from build123d import *

# Parameters (mm, degrees)
SKETCH_1_W          = 4.708553468
SKETCH_1_H          = 29.97466091
EXTRUDE_1_DEPTH     = 4.1
EXTRUDE_1_2_DEPTH   = 4.1
SKETCH_2_W          = 4.708553468
SKETCH_2_H          = 29.97466091
EXTRUDE_2_DEPTH     = 9
SKETCH_3_W          = 6
SKETCH_3_H          = 29.97466091
EXTRUDE_3_DEPTH     = 32.057569214
SKETCH_6_R          = 1
EXTRUDE_4_DEPTH     = 3
SKETCH_7_R          = 1.5
EXTRUDE_5_DEPTH     = 0.5
CUT_EXTRUDE_1_REACH = 33.926
SKETCH_9_W          = 32.057569214
SKETCH_9_H          = 5.97466091
EXTRUDE_6_DEPTH     = 2
SKETCH_12_W         = 4.708553468
SKETCH_12_H         = 13.1
EXTRUDE_7_DEPTH     = 2
SKETCH_13_W         = 32.057569214
SKETCH_13_H         = 6
CUT_EXTRUDE_3_DEPTH = 6.8
CUT_EXTRUDE_4_REACH = 35.242
SKETCH_14_W         = 3.528784607
SKETCH_14_H         = 10.5
CHAMFER_1_SIZE      = 2
CHAMFER_2_SIZE      = 0.5
CUT_EXTRUDE_5_REACH = 44.936
SKETCH_15_W         = 0.5
SKETCH_15_H         = 1
CHAMFER_3_SIZE      = 0.2
CHAMFER_4_SIZE      = 0.2
SKETCH_16_W         = 32.057569214
SKETCH_16_H         = 2
EXTRUDE_8_DEPTH     = 13.1
CUT_EXTRUDE_7_REACH = 43.372
SKETCH_18_W         = 32.057569214
SKETCH_18_H         = 2
EXTRUDE_9_DEPTH     = 7.1
CUT_EXTRUDE_8_DEPTH = 4


with BuildPart() as part:
    # Sketch 1 → Extrude 1 (new body)
    with BuildSketch(Plane.XY):
        with Locations((-18.383061341, 5.449009398)):
            Rectangle(SKETCH_1_W, SKETCH_1_H)
    extrude(amount=EXTRUDE_1_DEPTH)



with BuildPart() as body_2:
    # Sketch 1 → Extrude 1 2 (new body)
    with BuildSketch(Plane.XY):
        with Locations((18.383061341, 5.449009398)):
            Rectangle(SKETCH_1_W, SKETCH_1_H)
    extrude(amount=EXTRUDE_1_2_DEPTH)


with BuildPart() as part_1:
    add(part.part)

    add(body_2.part)  # Extrude 2 merges body 2
    # Sketch 2 → Extrude 2 (add)
    with BuildSketch(Plane.XY.offset(4.1)):
        with Locations((-18.383061341, 5.449009398)):
            Rectangle(SKETCH_2_W, SKETCH_2_H)
        with Locations((18.383061341, 5.449009398)):
            Rectangle(SKETCH_2_W, SKETCH_2_H)
    extrude(amount=EXTRUDE_2_DEPTH)

    # Sketch 3 → Extrude 3 (add)
    with BuildSketch(Plane.ZY.offset(-16.028784607)):
        with Locations((10.1, 5.449009398)):
            Rectangle(SKETCH_3_W, SKETCH_3_H)
    extrude(amount=EXTRUDE_3_DEPTH)

    # Sketch 6 → Extrude 4 (add)
    with BuildSketch(Plane.XY.offset(13.1)):
        with Locations((-10.5, 5.961678943)):
            Circle(SKETCH_6_R)
        with Locations((10.5, -7.538321057)):
            Circle(SKETCH_6_R)
        with Locations((-10.5, -7.538321057)):
            Circle(SKETCH_6_R)
        with Locations((10.5, 5.961678943)):
            Circle(SKETCH_6_R)
    extrude(amount=EXTRUDE_4_DEPTH)

    # Sketch 7 → Extrude 5 (add)
    with BuildSketch(Plane.XY.offset(13.1)):
        with Locations((-10.5, 5.961678943)):
            Circle(SKETCH_7_R)
        with Locations((-10.5, -7.538321057)):
            Circle(SKETCH_7_R)
        with Locations(Location((10.5, -7.538321057, 0), (0, 0, 180))):
            Circle(SKETCH_7_R)
        with Locations(Location((10.5, 5.961678943, 0), (0, 0, 180))):
            Circle(SKETCH_7_R)
    extrude(amount=EXTRUDE_5_DEPTH)

    # Sketch 9 → Cut-Extrude 1 (cut, up to next)
    with BuildSketch(Plane.XY.offset(13.1), mode=Mode.PRIVATE) as cut_extrude_1_sk1:
        with Locations((0, 17.449009398)):
            Rectangle(SKETCH_9_W, SKETCH_9_H)
    cut_extrude_1_tool1 = extrude(cut_extrude_1_sk1.sketch, amount=-CUT_EXTRUDE_1_REACH, mode=Mode.PRIVATE) & part_1.part
    add(cut_extrude_1_tool1.solids().sort_by_distance((0, 17.449009, 13.1))[0], mode=Mode.SUBTRACT)

    # Sketch 11 → Extrude 6 (add)
    with BuildSketch(Plane.XZ.offset(9.538321057)):
        Polygon((-20.737338075, 0), (-16.028784607, 0), (-16.028784607, 7.1), (16.028784607, 7.1), (16.028784607, 0), (20.737338075, 0), (20.737338075, 13.1), (-20.737338075, 13.1), align=None)
    extrude(amount=EXTRUDE_6_DEPTH)

    # Sketch 12 → Extrude 7 (add)
    with BuildSketch(Plane(origin=(0, 20.436339853, 0), x_dir=(1, 0, 0), z_dir=(0, 1, 0))):
        with Locations((18.383061341, -6.55)):
            Rectangle(SKETCH_12_W, SKETCH_12_H)
        with Locations((-18.383061341, -6.55)):
            Rectangle(SKETCH_12_W, SKETCH_12_H)
    extrude(amount=EXTRUDE_7_DEPTH)

    # Sketch 13 → Cut-Extrude 3 (cut)
    with BuildSketch(Plane(origin=(0, 14.461678943, 0), x_dir=(1, 0, 0), z_dir=(0, 1, 0))):
        with Locations((0, -10.1)):
            Rectangle(SKETCH_13_W, SKETCH_13_H)
    extrude(amount=-CUT_EXTRUDE_3_DEPTH, mode=Mode.SUBTRACT)

    # Sketch 14 → Cut-Extrude 4 (cut, up to next)
    with BuildSketch(Plane.XY.offset(13.1), mode=Mode.PRIVATE) as cut_extrude_4_sk1:
        with Locations((-14.264392304, -0.788321057)):
            Rectangle(SKETCH_14_W, SKETCH_14_H)
    cut_extrude_4_tool1 = extrude(cut_extrude_4_sk1.sketch, amount=-CUT_EXTRUDE_4_REACH, mode=Mode.PRIVATE) & part_1.part
    # Sketch 14 → Cut-Extrude 4 (cut, up to next)
    with BuildSketch(Plane.XY.offset(13.1), mode=Mode.PRIVATE) as cut_extrude_4_sk2:
        with Locations((14.264392304, -0.788321057)):
            Rectangle(SKETCH_14_W, SKETCH_14_H)
    cut_extrude_4_tool2 = extrude(cut_extrude_4_sk2.sketch, amount=-CUT_EXTRUDE_4_REACH, mode=Mode.PRIVATE) & part_1.part
    add(cut_extrude_4_tool1.solids().sort_by_distance((-14.264392, -0.788321, 13.1))[0], mode=Mode.SUBTRACT)
    add(cut_extrude_4_tool2.solids().sort_by_distance((14.264392, -0.788321, 13.1))[0], mode=Mode.SUBTRACT)

    # Chamfer 1
    chamfer_1_edges = [part_1.edges().sort_by_distance(p)[0] for p in [
        (-20.737338075, 5.449009398, 13.1),
        (20.737338075, 5.449009398, 13.1),
    ]]
    chamfer(chamfer_1_edges, length=CHAMFER_1_SIZE)

    # Chamfer 2
    chamfer_2_edges = [part_1.edges().sort_by_distance(p)[0] for p in [
        (16.028784607, 7.661678943, 10.1),
        (-16.028784607, 7.661678943, 10.1),
        (-16.028784607, -6.038321057, 10.1),
        (-12.5, 4.461678943, 10.1),
        (-12.5, -6.038321057, 10.1),
        (-16.028784607, 4.461678943, 10.1),
        (16.028784607, 4.461678943, 10.1),
        (12.5, 4.461678943, 10.1),
        (16.028784607, -6.038321057, 10.1),
        (12.5, -6.038321057, 10.1),
    ]]
    chamfer(chamfer_2_edges, length=CHAMFER_2_SIZE)

    # Sketch 15 → Cut-Extrude 5 (cut, up to next)
    with BuildSketch(Plane.XZ.offset(11.538321057), mode=Mode.PRIVATE) as cut_extrude_5_sk1:
        with Locations((-20.487338075, 5.05)):
            Rectangle(SKETCH_15_W, SKETCH_15_H)
    cut_extrude_5_tool1 = extrude(cut_extrude_5_sk1.sketch, amount=-CUT_EXTRUDE_5_REACH, mode=Mode.PRIVATE) & part_1.part
    # Sketch 15 → Cut-Extrude 5 (cut, up to next)
    with BuildSketch(Plane.XZ.offset(11.538321057), mode=Mode.PRIVATE) as cut_extrude_5_sk2:
        with Locations((-20.487338075, 3.55)):
            Rectangle(SKETCH_15_W, SKETCH_15_H)
    cut_extrude_5_tool2 = extrude(cut_extrude_5_sk2.sketch, amount=-CUT_EXTRUDE_5_REACH, mode=Mode.PRIVATE) & part_1.part
    # Sketch 15 → Cut-Extrude 5 (cut, up to next)
    with BuildSketch(Plane.XZ.offset(11.538321057), mode=Mode.PRIVATE) as cut_extrude_5_sk3:
        with Locations((-20.487338075, 2.05)):
            Rectangle(SKETCH_15_W, SKETCH_15_H)
    cut_extrude_5_tool3 = extrude(cut_extrude_5_sk3.sketch, amount=-CUT_EXTRUDE_5_REACH, mode=Mode.PRIVATE) & part_1.part
    # Sketch 15 → Cut-Extrude 5 (cut, up to next)
    with BuildSketch(Plane.XZ.offset(11.538321057), mode=Mode.PRIVATE) as cut_extrude_5_sk4:
        with Locations((-20.487338075, 6.55)):
            Rectangle(SKETCH_15_W, SKETCH_15_H)
    cut_extrude_5_tool4 = extrude(cut_extrude_5_sk4.sketch, amount=-CUT_EXTRUDE_5_REACH, mode=Mode.PRIVATE) & part_1.part
    # Sketch 15 → Cut-Extrude 5 (cut, up to next)
    with BuildSketch(Plane.XZ.offset(11.538321057), mode=Mode.PRIVATE) as cut_extrude_5_sk5:
        with Locations((20.487338075, 5.55)):
            Rectangle(SKETCH_15_W, SKETCH_15_H)
    cut_extrude_5_tool5 = extrude(cut_extrude_5_sk5.sketch, amount=-CUT_EXTRUDE_5_REACH, mode=Mode.PRIVATE) & part_1.part
    # Sketch 15 → Cut-Extrude 5 (cut, up to next)
    with BuildSketch(Plane.XZ.offset(11.538321057), mode=Mode.PRIVATE) as cut_extrude_5_sk6:
        with Locations((20.487338075, 1.05)):
            Rectangle(SKETCH_15_W, SKETCH_15_H)
    cut_extrude_5_tool6 = extrude(cut_extrude_5_sk6.sketch, amount=-CUT_EXTRUDE_5_REACH, mode=Mode.PRIVATE) & part_1.part
    # Sketch 15 → Cut-Extrude 5 (cut, up to next)
    with BuildSketch(Plane.XZ.offset(11.538321057), mode=Mode.PRIVATE) as cut_extrude_5_sk7:
        with Locations((20.487338075, 2.55)):
            Rectangle(SKETCH_15_W, SKETCH_15_H)
    cut_extrude_5_tool7 = extrude(cut_extrude_5_sk7.sketch, amount=-CUT_EXTRUDE_5_REACH, mode=Mode.PRIVATE) & part_1.part
    # Sketch 15 → Cut-Extrude 5 (cut, up to next)
    with BuildSketch(Plane.XZ.offset(11.538321057), mode=Mode.PRIVATE) as cut_extrude_5_sk8:
        with Locations((20.487338075, 4.05)):
            Rectangle(SKETCH_15_W, SKETCH_15_H)
    cut_extrude_5_tool8 = extrude(cut_extrude_5_sk8.sketch, amount=-CUT_EXTRUDE_5_REACH, mode=Mode.PRIVATE) & part_1.part
    add(cut_extrude_5_tool1.solids().sort_by_distance((-20.487338, -11.538321, 5.05))[0], mode=Mode.SUBTRACT)
    add(cut_extrude_5_tool2.solids().sort_by_distance((-20.487338, -11.538321, 3.55))[0], mode=Mode.SUBTRACT)
    add(cut_extrude_5_tool3.solids().sort_by_distance((-20.487338, -11.538321, 2.05))[0], mode=Mode.SUBTRACT)
    add(cut_extrude_5_tool4.solids().sort_by_distance((-20.487338, -11.538321, 6.55))[0], mode=Mode.SUBTRACT)
    add(cut_extrude_5_tool5.solids().sort_by_distance((20.487338, -11.538321, 5.55))[0], mode=Mode.SUBTRACT)
    add(cut_extrude_5_tool6.solids().sort_by_distance((20.487338, -11.538321, 1.05))[0], mode=Mode.SUBTRACT)
    add(cut_extrude_5_tool7.solids().sort_by_distance((20.487338, -11.538321, 2.55))[0], mode=Mode.SUBTRACT)
    add(cut_extrude_5_tool8.solids().sort_by_distance((20.487338, -11.538321, 4.05))[0], mode=Mode.SUBTRACT)

    # Chamfer 3
    chamfer_3_edges = [part_1.edges().sort_by_distance(p)[0] for p in [
        (-20.237338075, 5.449009398, 4.05),
        (-20.237338075, 5.449009398, 3.05),
        (-20.237338075, 5.449009398, 2.55),
        (-20.237338075, 5.449009398, 1.55),
        (-20.237338075, 5.449009398, 7.05),
        (-20.237338075, 5.449009398, 6.05),
        (-20.237338075, 5.449009398, 5.55),
        (-20.237338075, 5.449009398, 4.55),
    ]]
    chamfer(chamfer_3_edges, length=CHAMFER_3_SIZE)

    # Chamfer 4
    chamfer_4_edges = [part_1.edges().sort_by_distance(p)[0] for p in [
        (20.237338075, 5.449009398, 6.05),
        (20.237338075, 5.449009398, 5.05),
        (20.237338075, 5.449009398, 1.55),
        (20.237338075, 5.449009398, 0.55),
        (20.237338075, 5.449009398, 3.05),
        (20.237338075, 5.449009398, 2.05),
        (20.237338075, 5.449009398, 4.55),
        (20.237338075, 5.449009398, 3.55),
    ]]
    chamfer(chamfer_4_edges, length=CHAMFER_4_SIZE)

    # Sketch 16 → Extrude 8 (add)
    with BuildSketch(Plane(origin=(0, 0, 0), x_dir=(-1, 0, 0), z_dir=(0, 0, -1))):
        with Locations((0, 21.436339853)):
            Rectangle(SKETCH_16_W, SKETCH_16_H)
    extrude(amount=-EXTRUDE_8_DEPTH)

    # Sketch 17 → Cut-Extrude 7 (cut, up to next)
    with BuildSketch(Plane.XZ.offset(-20.436339853), mode=Mode.PRIVATE) as cut_extrude_7_sk1:
        with BuildLine():
            Line((4.465561881, 1.229756424), (4.470622966, 1.343469934))
            Line((4.470622966, 1.343469934), (4.470622966, 1.943469934))
            add(Edge.make_bspline(
                [(4.470622966, 1.943469934), (4.470622966, 3.223469934), (3.190622966, 3.223469934)],
                knots=[1.814608209, 1.814608209, 1.814608209, 3.385404536, 3.385404536, 3.385404536], degree=2, weights=[1, 0.707106781, 1]))
            Line((3.190622966, 3.223469934), (-3.189377034, 3.223469934))
            ThreePointArc((-3.189377034, 3.223469934), (-4.094473714, 2.848566614), (-4.469377034, 1.943469934))
            Line((-4.469377034, 1.943469934), (-4.469377034, 1.343469934))
            Line((-4.469377034, 1.343469934), (-4.489171494, 5.5e-08))
            Line((-4.489171494, 5.5e-08), (4.410828707, 4e-09))
            Line((4.410828707, 4e-09), (4.465561881, 1.229756424))
        make_face()
    cut_extrude_7_tool1 = extrude(cut_extrude_7_sk1.sketch, amount=-CUT_EXTRUDE_7_REACH, mode=Mode.PRIVATE) & part_1.part
    add(cut_extrude_7_tool1.solids().sort_by_distance((-0.00786, 20.43634, 1.579655))[0], mode=Mode.SUBTRACT)

    # Sketch 18 → Extrude 9 (add)
    with BuildSketch(Plane(origin=(0, 0, 7.1), x_dir=(-1, 0, 0), z_dir=(0, 0, -1))):
        with Locations((0, -10.538321057)):
            Rectangle(SKETCH_18_W, SKETCH_18_H)
    extrude(amount=EXTRUDE_9_DEPTH)

    # Sketch 19 → Cut-Extrude 8 (cut)
    with BuildSketch(Plane(origin=(0, 0, 7.1), x_dir=(-1, 0, 0), z_dir=(0, 0, -1))):
        Polygon((-16.028784607, -5.538321057), (-16.028784607, -9.538321057), (16.028784607, -9.538321057), (16.028784607, -5.538321057), (15.528784607, -6.038321057), (13, -6.038321057), (12.5, -5.538321057), (12.5, 3.961678943), (13, 4.461678943), (15.528784607, 4.461678943), (16.028784607, 3.961678943), (16.028784607, 8.161678943), (15.528784607, 7.661678943), (-15.528784607, 7.661678943), (-16.028784607, 8.161678943), (-16.028784607, 3.961678943), (-15.528784607, 4.461678943), (-13, 4.461678943), (-12.5, 3.961678943), (-12.5, -5.538321057), (-13, -6.038321057), (-15.528784607, -6.038321057), align=None)
    extrude(amount=-CUT_EXTRUDE_8_DEPTH, mode=Mode.SUBTRACT)


solid = part_1.part
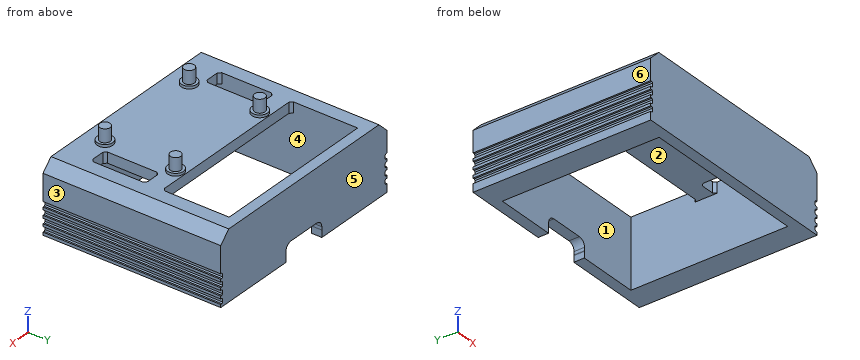
Geometry: final body of the model. Coordinates: model frame, mm. Face numbers are marked on the shaded views. A direction names the side the tool comes from. Round coordinates to 2 decimals unless told otherwise and drop trailing zeros. Order: outer loops, then holes, each group sorted by start corner. A loop starts at its lowest first (then second) coordinate and runs counter-clockwise, first axis right, second up. Notation, with made-up numbers: (44, 67.25) - (100, 67.25) arc R25 cw to (100, 82.25) - close; hole circle Ø2 at (39.5, 17.5). An arc over 180 degrees is marked (long way). Write each question's results on one line, items separated by ' | '.
Item 1: Section A-A, the plane x = 7. Return the cut outline in (y, z), and give its area (3 significant figures).
Completed:
outline: (-11.54, 0) - (-9.54, 0) - (-9.54, 11.1) - (7.66, 11.1) - (7.66, 13.1) - (-11.54, 13.1) - close; (20.44, 0) - (22.44, 0) - (22.44, 13.1) - (20.44, 13.1) - close | area: 86.8 mm^2
Item 2: Reachability of the marked faces 1, 2 and 3 from +Z, -Z, +X, -X, +Y, -Y: full face, straight path, thin tool, end or side. Return the list, or none.
Completed:
face 1: +Z, -Z | face 2: -Z | face 3: +Z, -Z, +X, +Y, -Y
Item 3: Section D-D, the plane x = 17.5. Return the cut outline in (y, z).
Completed:
outline: (-11.54, 0) - (22.44, 0) - (22.44, 13.1) - (-11.54, 13.1) - close
Item 4: Section B-B, the plane z = 8.5. Return the cut outline in (x, y), and give its area (3 significant figures).
Completed:
outline: (-20.74, -11.54) - (20.74, -11.54) - (20.74, 22.44) - (-20.74, 22.44) - close; hole (-16.03, -9.54) - (16.03, -9.54) - (16.03, 20.44) - (-16.03, 20.44) - close | area: 448 mm^2
Item 5: Section C-C, the plane y = 2.5. State how many separate pieces and enclosed holes the cut face has, and give its area (3 significant figures).
Completed:
separate pieces: 3 | enclosed holes: 0 | area: 166 mm^2
Item 6: Mould query, pull axis X, two halves, no side actions, for the marked faces 4, 5 and 6. Classes: pulls with the +X half, pulls with the -X half, needs draft (parallel to the pull), parting line crosses it, or undercut.
Completed:
face 4: undercut | face 5: needs draft | face 6: pulls with the -X half
Item 7: First-contact query: pin 1 Ø5 at (x, y) = (11, 17) entering from +Z; pin 2 Ø1 at (x, y) = (10.5, -2.5) entering from -Z; pin 3 Ø3 at (x, y) = (5.5, 4) entering from +Z. Flat tips, straight axial feed; report the tip coordinate or a pass-through.
Completed:
pin 1: through | pin 2: z = 11.1 | pin 3: z = 13.1
Item 8: Material intervals for line 1 along X through (y, z) = (15.5, 9.5); line 2 along X through (y, z) = (6.5, 6.5); line 3 along Y through (x, z) = (2.5, 8.75), sorted ascending. Write a range as [from, to].
Completed:
line 1: [-20.74, -16.03], [16.03, 20.74] | line 2: [-20.24, -16.03], [16.03, 20.74] | line 3: [-11.54, -9.54], [20.44, 22.44]
